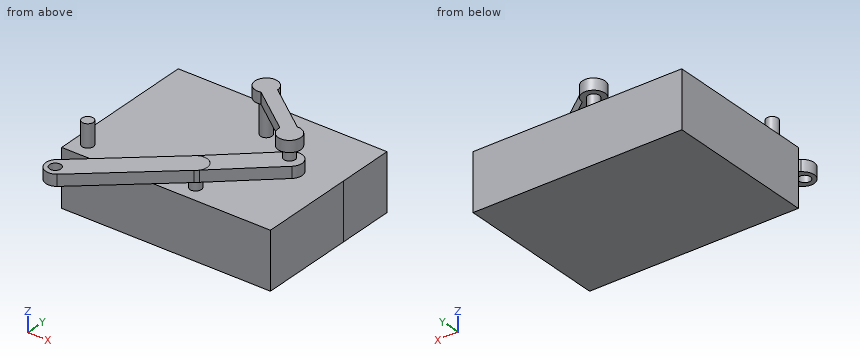
Autodesk Inventor part; units mm, degrees
ref_plane "YZ Plane" through (0, 0, 0) normal (1, 0, 0) x (0, 1, 0)
ref_plane "XZ Plane" through (0, 0, 0) normal (0, 1, 0) x (-1, 0, 0)
ref_plane "XY Plane" through (0, 0, 0) normal (0, 0, 1) x (1, 0, 0)
sketch "Эскиз1" plane through (0, 0, 0) normal (0, 0, 1) x (1, 0, 0)
  line L0 (10.0582, -8.8009) -> (-16.8718, -8.8009)
  line L1 (-16.8718, -8.8009) -> (-16.8718, 8.0709)
  line L2 (-16.8718, 8.0709) -> (10.0582, 8.0709)
  line L3 (10.0582, 8.0709) -> (10.0582, -8.8009)
  point P0 (0, 0)
extrude "Выдавливание1" add sketch "Эскиз1" along normal blind 10
sketch "Эскиз2" plane through (0, 0, 10) normal (0, 0, 1) x (1, 0, 0)
  circle A0 centre (4.6641, -5.9619) radius 1
  circle A1 centre (-14.4383, -5.9619) radius 1
  point P0 (0, 0)
  dimension "d2" = 2
  dimension "d3" = 2
extrude "Выдавливание2" add sketch "Эскиз2" along normal blind 2
sketch "Эскиз3" plane through (4.6641, -5.9619, 12) normal (0, 0, 1) x (1, 0, 0)
  circle A0 centre (0, 0) radius 1
  circle A1 centre (0, 0) radius 2
  circle A2 centre (-14.7836, -12.664) radius 2
  line L0 (-1.2061, 1.5954) -> (-15.8126, -10.949)
  line L1 (-13.5836, -14.264) -> (1.0265, -1.7165)
  point P0 (-4.6641, 5.9619)
  dimension "d6" = 4
  dimension "d7" = 4
extrude "Выдавливание3" add sketch "Эскиз3" along normal blind 2
sketch "Эскиз4" plane through (-14.4383, -5.9619, 12) normal (0, 0, 1) x (1, 0, 0)
  circle A0 centre (0, 0) radius 1
  point P0 (14.4383, 5.9619)
extrude "Выдавливание4" add sketch "Эскиз4" along normal blind 4
sketch "Эскиз5" plane through (4.6641, -5.9619, 14) normal (0, 0, 1) x (1, 0, 0)
  circle A0 centre (-10.7969, -8.6603) radius 1
  point P0 (-4.6641, 5.9619)
  dimension "d12" = 2
extrude "Выдавливание5" add sketch "Эскиз5" along normal blind 2
sketch "Эскиз6" plane through (4.6641, -5.9619, 14) normal (0, 0, 1) x (1, 0, 0)
  circle A0 centre (-15.0265, -12.7992) radius 1
  point P0 (-4.6641, 5.9619)
  dimension "d15" = 2
extrude "Выдавливание6" cut sketch "Эскиз6" against normal blind 10
sketch "Эскиз7" plane through (-14.4383, -5.9619, 16) normal (0, 0, 1) x (1, 0, 0)
  circle A0 centre (0, 0) radius 2
  circle A1 centre (8.3055, -8.6603) radius 1
  circle A2 centre (8.3055, -8.6603) radius 2
  line L0 (7.3055, -6.9282) -> (1.7093, -1.0384)
  line L1 (6.6268, -7.5731) -> (1.0492, -1.7027)
  point P0 (14.4383, 5.9619)
  dimension "d18" = 4
  dimension "d19" = 4
extrude "Выдавливание7" add sketch "Эскиз7" along normal blind 2 contours A0 | A0 L0 A2 L1 | A2 | A1
sketch "Эскиз8" plane through (-14.4383, -5.9619, 18) normal (0, 0, 1) x (1, 0, 0)
  circle A0 centre (0, 0) radius 1
  point P0 (14.4383, 5.9619)
extrude "Выдавливание8" cut sketch "Эскиз8" against normal blind 1
chamfer "Фаска1" distance 0.3 angle 45 4 edges at (-9.9309, -9.9452, 18) (-9.9309, -9.9452, 16) (-10.6004, -10.5998, 16) (-10.6004, -10.5998, 18)
sketch "Эскиз9" plane through (-14.4383, -5.9619, 18) normal (0, 0, 1) x (1, 0, 0)
  line L0 (-16.7765, 10.1097) -> (30.4978, 10.1097)
  line L1 (30.4978, 10.1097) -> (30.4978, -12.7564)
  line L2 (30.4978, -12.7564) -> (-16.7765, -12.7564)
  line L3 (-16.7765, -12.7564) -> (-16.7765, 10.1097)
  point P0 (14.4383, 5.9619)
extrude "Выдавливание9" cut sketch "Эскиз9" against normal blind 4
sketch "Эскиз10" plane through (10.0582, -8.8009, 0) normal (1, 0, 0) x (0, 0, -1)
  line L0 (0, 0) -> (0, 16.8718)
  line L1 (-10, 0) -> (-10, 16.8718)
  line L2 (0, 0) -> (-10, 0)
  line L3 (-10, 0) -> (-10, 16.8718)
  line L4 (-10, 16.8718) -> (0, 16.8718)
  line L5 (0, 16.8718) -> (0, 0)
  point P0 (0, 8.8009)
extrude "Выдавливание10" add sketch "Эскиз10" along normal blind 10
sketch "Эскиз11" plane through (4.6641, -5.9619, 14) normal (0, 0, 1) x (1, 0, 0)
  circle A0 centre (9.9064, 8.993) radius 2
  arc A1 (1.0265, -1.7165) -> (-1.2061, 1.5954) centre (0, 0) ccw
  line L0 (8.4408, 10.3539) -> (-1.2061, 1.5954)
  line L1 (-1.2061, 1.5954) -> (1.0265, -1.7165)
  line L2 (1.0265, -1.7165) -> (11.2465, 7.5083)
  point P0 (-4.6641, 5.9619)
  point P1 (1.6027, -1.1964)
  dimension "d31" = 4
extrude "Выдавливание11" add sketch "Эскиз11" against normal blind 2 contours A0 | A0 L2 A1 L0
sketch "Эскиз12" plane through (-16.8718, 8.0709, 10) normal (0, 1, 0) x (1, 0, 0)
  line L0 (0, 10) -> (36.9299, 10)
  line L1 (0, 0) -> (36.9299, 0)
  line L2 (0, 10) -> (36.9299, 10)
  line L3 (36.9299, 10) -> (36.9299, 0)
  line L4 (36.9299, 0) -> (0, 0)
  line L5 (0, 0) -> (0, 10)
  point P0 (16.8718, 10)
extrude "Выдавливание12" add sketch "Эскиз12" along normal blind 10
sketch "Эскиз13" plane through (0, 0, 10) normal (0, 0, 1) x (1, 0, 0)
  circle A0 centre (3.7224, 11.5394) radius 1
  point P0 (0, 0)
  dimension "d36" = 2
extrude "Выдавливание13" add sketch "Эскиз13" along normal blind 6
sketch "Эскиз14" plane through (4.6641, -5.9619, 14) normal (0, 0, 1) x (1, 0, 0)
  circle A0 centre (9.5274, 9.2057) radius 1
  point P0 (-4.6641, 5.9619)
  dimension "d39" = 2
extrude "Выдавливание14" add sketch "Эскиз14" along normal blind 2
sketch "Эскиз15" plane through (3.7224, 11.5394, 16) normal (0, 0, 1) x (1, 0, 0)
  circle A0 centre (0, 0) radius 1
  circle A1 centre (0, 0) radius 2
  circle A2 centre (10.469, -8.2956) radius 1
  circle A3 centre (10.469, -8.2956) radius 2
  line L0 (10.314, -6.3017) -> (2, 0)
  line L1 (9.3825, -7.1474) -> (-0.2644, -15.9059)
  line L2 (8.4993, -7.9493) -> (0.5405, -1.9256)
  point P0 (-3.7224, -11.5394)
  dimension "d42" = 4
  dimension "d43" = 4
extrude "Выдавливание15" add sketch "Эскиз15" along normal blind 2 contours A0 | A1 | L0 A3 L2 A1 | A3 | A2
For this review, take the finished solid that the model builds, in its own axes (mm). Coordinates: 2 decimals unless noted, no trailing zeros. Write each loop counter-clockwise with the first axis right and the second up, starting at its lowest first coordinate (ties: lowest second). Pieces come first, ordered by that corner, then holes. Notation, with made-up numbers: (12, 67.5) - (44, 67.5) arc R14 cw to (44, 90.5) - close; hole circle Ø7 at (34.5, -17). An arc over 180 degrees is marked (long way). Put each result on its own line as item: value.
1. Add section B-B, the plane x = 10. Give the boundary of the cut face in (y, z).
Values found:
outline: (-8.8, 0) - (18.07, 0) - (18.07, 10) - (-8.8, 10) - close; (-3.79, 12) - (1.57, 12) - (1.57, 14) - (-3.79, 14) - close; (5.27, 16) - (8.3, 16) - (8.3, 18) - (5.27, 18) - close
2. Wall thickness on probe 1 along Z at (x, y) = (9.5, -1); probe 2 along Y at (x, z) = (-1.5, 9); probe 3 along Z at (x, y) = (-0.5, -5): over which ranges is each line inside the solid? List them lowest first.
Values found:
probe 1: 0 to 10, 12 to 14
probe 2: -8.8 to 18.07
probe 3: 0 to 10
3. For pin 1 (1.6 mm diameter, centred on x = -15, y = -5.5, fed in from +Z); pin 2 (10 mm diameter, centred on x = 0, z = 16, fed in from +Y); pin 3 (1.5 mm diameter, centred on x = 2.5, y = 3.5, fed in from +Z), all flat-tipped, find the tip position at first contact; note any pin that passes through.
Values found:
pin 1: z = 14
pin 2: y = 13.54
pin 3: z = 10
4. Add section A-A, the plane y = 13. Give the boundary of the cut face in (x, z), then the cut area to 3 significant figures.
Values found:
outline: (-16.87, 0) - (20.06, 0) - (20.06, 10) - (-16.87, 10) - close; (2.36, 16) - (5.09, 16) - (5.09, 18) - (2.36, 18) - close
area: 375 mm²
5. Add section D-D, the plane x = -0.5. Give the boundary of the cut face in (y, z), then the cut area to 3 significant figures.
Values found:
outline: (-13, 12) - (-7.77, 12) - (-7.77, 14) - (-13, 14) - close; (-8.8, 0) - (18.07, 0) - (18.07, 10) - (-8.8, 10) - close
area: 279 mm²
